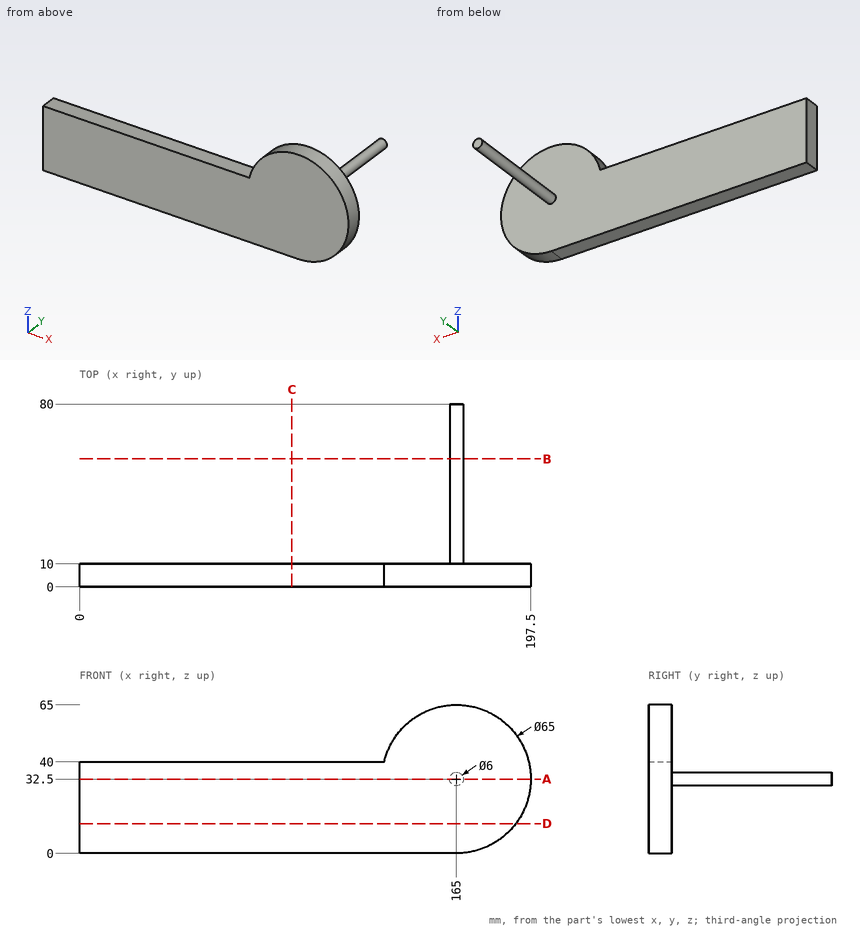
Input: dimensioned drawing with shaded views. Units: mm. Origin: part minimum x, y, z. Coordinates: 2 decimals unless noted, no trailing zeros. Write each loop counter-clockwise with the first axis right and the second up, starting at its lowest first coordinate (ties: lowest second). Pieces come first, ordered by that corner, then holes. Notation, with made-up numbers: M 25.5,26.25 L 75.5,26.25 A12 ccw 75.5,35.25 Z; hole C -12.75,74.5 d4. An arc over 180 degrees is marked long. Use a Markdown table: item, result.
1) Ray query, L1, parallel to Y at x = 149, z = 18; L2, parallel to Z at x = 17, y = 5.5; L3, parallel to X at y = 25, z = 32.5. Return the intervals inside material, ascending.
Conclusion:
| item | result |
|---|---|
| L1 | y = 0 to 10 |
| L2 | z = 0 to 40 |
| L3 | x = 162 to 168 |
2) Section B-B, the plane y = 56. Output: boundary loops of the cut face in (x, z).
Conclusion:
| item | result |
|---|---|
| outline | C 165,32.5 d6 |
3) Section C-C, the plane x = 93. Output: boundary loops of the cut face in (y, z).
Conclusion:
| item | result |
|---|---|
| outline | M 0,0 L 10,0 L 10,40 L 0,40 Z |
4) Section D-D, the plane z = 13. Output: boundary loops of the cut face in (x, y).
Conclusion:
| item | result |
|---|---|
| outline | M 0,0 L 191,0 L 191,10 L 0,10 Z |
5) First-contact query: pin 1 Ø5 at (x, y) = (34, 5) entering from +Z; pin 2 Ø2 at (x, z) = (175, 57.5) entering from -Y; pin 3 Ø1 at (x, z) = (120, 28.5) entering from +Y; pin 4 Ø1 at (y, z) = (51.5, 30.5) entering from +X. Flat tips, straight axial feed; report the tip coordinate or a pass-through.
Conclusion:
| item | result |
|---|---|
| pin 1 | stops at z = 40 |
| pin 2 | stops at y = 0 |
| pin 3 | stops at y = 10 |
| pin 4 | stops at x = 167.6 |
6) Section A-A, the plane z = 32.5. Output: boundary loops of the cut face in (x, y).
Conclusion:
| item | result |
|---|---|
| outline | M 0,0 L 197.5,0 L 197.5,10 L 168,10 L 168,80 L 162,80 L 162,10 L 0,10 Z |
